Check sheet for the modelled part. Datum: model origin and axes. Units: mm. A direction names the side the tool comes from. Give positions to 0.01 mm unless a question says otherwise; leave off trailing zeros. Order: outer loops, then holes, each group sorted by start corner. A loop starts at its lowest first (then second) coordinate and runs counter-clockwise, first axis right, second up. Notation, with made-up numbers: (44, 43.5) -> (67, 43.5) arc R13 cw to (67, 67.5) -> close; hole circle Ø4 at (70.25, 5.25). An arc over 180 degrees is marked (long way). One line per question, with ' | ' between items.
Autodesk Inventor part; units mm, degrees
ref_plane "YZ Plane" through (0, 0, 0) normal (1, 0, 0) x (0, 1, 0)
ref_plane "XZ Plane" through (0, 0, 0) normal (0, 1, 0) x (-1, 0, 0)
ref_plane "XY Plane" through (0, 0, 0) normal (0, 0, 1) x (1, 0, 0)
sketch "Sketch1" plane through (0, 0, 0) normal (0, 0, 1) x (1, 0, 0)
  line L0 (0, 0) -> (0, 63.5)
  line L1 (0, 63.5) -> (203.2, 63.5)
  line L2 (203.2, 63.5) -> (203.2, 0)
  line L3 (0, 0) -> (203.2, 0)
  dimension "d0" = 63.5
  dimension "d1" = 203.2
extrude "Extrusion1" add sketch "Sketch1" along normal blind 12.7
sketch "Sketch2" plane through (0, 0, 12.7) normal (0, 0, 1) x (1, 0, 0)
  line L0 (0, 63.5) -> (0, 0)
  line L1 (203.2, 0) -> (203.2, 63.5)
  line L2 (0, 57.15) -> (203.2, 57.15)
  line L3 (203.2, 57.15) -> (203.2, 6.35)
  line L4 (203.2, 6.35) -> (0, 6.35)
  line L5 (0, 6.35) -> (0, 57.15)
  line L6 (0, 63.5) -> (203.2, 63.5)
  line L7 (203.2, 0) -> (0, 0)
  dimension "d4" = 6.35
  dimension "d5" = 6.35
extrude "Extrusion2" cut sketch "Sketch2" against normal blind 6.35 contours L2 L1 L4 L0
sketch "Sketch3" plane through (0, 0, 6.35) normal (0, 0, 1) x (1, 0, 0)
  arc A0 (0, 0) -> (203.2, 0) centre (101.6, 50.8) ccw
  line L0 (0, 0) -> (203.2, 0)
  dimension "d8" = 50.8
extrude "Extrusion3" add sketch "Sketch3" along normal mid plane 12.7
sketch "Sketch4" plane through (0, 0, 6.35) normal (0, 0, 1) x (1, 0, 0)
  circle A0 centre (101.6, 31.75) radius 11.1125
  circle A1 centre (101.6, 24.13) radius 11.1125
  line L0 (203.2, 57.15) -> (203.2, 6.35)
  line L1 (0, 57.15) -> (203.2, 57.15)
  line L2 (90.4875, 31.75) -> (90.4875, 24.13)
  line L3 (112.7125, 31.75) -> (112.7125, 24.13)
  point P0 (0, 0)
  dimension "d11" = 101.6
  dimension "d12" = 101.6
  dimension "d13" = 22.225
  dimension "d14" = 7.62
  dimension "d15" = 22.225
  dimension "d16" = 25.4
extrude "Extrusion4" cut sketch "Sketch4" against normal blind 12.7
properties part number "C11_ZP_middle wheel plate"
Q1. Section check D-D (y = 48.5). Enter the section's corners in (x, z).
Result sheet:
outline: (0, 0) -> (203.2, 0) -> (203.2, 6.35) -> (0, 6.35) -> close
Q2. Section check C-C (x = 127). Enter the section's corners in (y, z), and give its area (3 significant figures).
Result sheet:
outline: (-59.92, 0) -> (63.5, 0) -> (63.5, 12.7) -> (57.15, 12.7) -> (57.15, 6.35) -> (6.35, 6.35) -> (6.35, 12.7) -> (-59.92, 12.7) -> close | area: 1,240 mm2
Q3. Access from +Z, -Z, +X, -X, +Y, -Y to the whole of each face (thin tool, end or side, straight path). Record for faces 1 (the face through (100, 60, 12.7)), 2 (the face through (100, 43, 6.35)), 3 (the face through (90.488, 28, 3)).
Result sheet:
face 1: +Z, +X, -X, +Y, -Y | face 2: +Z, +X, -X | face 3: +Z, -Z
Q4. Section check B-B (x = 101.6). Enter the section's corners in (y, z), and give its area (3 significant figures).
Result sheet:
outline: (-62.79, 0) -> (13.02, 0) -> (13.02, 6.35) -> (6.35, 6.35) -> (6.35, 12.7) -> (-62.79, 12.7) -> close; (42.86, 0) -> (63.5, 0) -> (63.5, 12.7) -> (57.15, 12.7) -> (57.15, 6.35) -> (42.86, 6.35) -> close | area: 1,090 mm2
Q5. Mould release check, pull along X, two halves, no side actions. Record for faces 4 (the face through (100, -20, 12.7)), 5 (the face through (0, 31, 5)), 6 (the face through (112.712, 28, 3)): pulls with the +X half, pulls with the -X half, needs draft (parallel to the pull), parting line crosses it, or undercut.
Result sheet:
face 4: needs draft | face 5: pulls with the -X half | face 6: undercut
Q6. Depth check by flat-ended pin: pin 1 Ø2 at (x, y) = (130.5, 38.5) entering from +Z; pin 2 Ø3 at (x, z) = (113.5, 10.5) entering from -Y; pin 3 Ø5 at (y, z) = (-33.5, 2) entering from +X. Enter the tip coordinate at first touch or a pass-through.
Result sheet:
pin 1: stops at z = 6.35 | pin 2: stops at y = -62.32 | pin 3: stops at x = 180.42
Q7. Thickness scan on line 1 (Z direction, x = 119, y = 8); line 2 (Y direction, x = 53.5, z = 10); line 3 (Y direction, x = 91.5, z = 6.75). Record the ranges inside material, lowest first.
Result sheet:
line 1: z = 0 to 6.35 | line 2: y = -52.11 to 6.35, 57.15 to 63.5 | line 3: y = -62.34 to 6.35, 57.15 to 63.5
